from build123d import *

# Parameters (mm, degrees)
SKETCH1_W           = 47
SKETCH1_H           = 17
BOSS_EXTRUDE1_DEPTH = 23
SKETCH2_W           = 4
SKETCH2_H           = 18
CUT_EXTRUDE1_DEPTH  = 38.016888038
SKETCH3_R           = 2
CUT_EXTRUDE2_DEPTH  = 8


with BuildPart() as part:
    # Sketch1 → Boss-Extrude1 (new body)
    with BuildSketch(Plane(origin=(0, 0, 0), x_dir=(1, 0, 0), z_dir=(0, 1, 0))):
        Rectangle(SKETCH1_W, SKETCH1_H)
    extrude(amount=BOSS_EXTRUDE1_DEPTH)

    # Sketch2 → Cut-Extrude1 (cut, through all)
    with BuildSketch(Plane.XY.offset(8.5)):
        with Locations((-20.70480001, 14)):
            Rectangle(SKETCH2_W, SKETCH2_H)
        with Locations((-15.55480001, 14)):
            Rectangle(SKETCH2_W, SKETCH2_H)
        with Locations((-10.40480001, 14)):
            Rectangle(SKETCH2_W, SKETCH2_H)
        with Locations((-5.25480001, 14)):
            Rectangle(SKETCH2_W, SKETCH2_H)
        with Locations((-0.10480001, 14)):
            Rectangle(SKETCH2_W, SKETCH2_H)
        with Locations((5.04519999, 14)):
            Rectangle(SKETCH2_W, SKETCH2_H)
        with Locations((10.19519999, 14)):
            Rectangle(SKETCH2_W, SKETCH2_H)
        with Locations((15.34519999, 14)):
            Rectangle(SKETCH2_W, SKETCH2_H)
        with Locations((20.49519999, 14)):
            Rectangle(SKETCH2_W, SKETCH2_H)
    extrude(amount=-CUT_EXTRUDE1_DEPTH, mode=Mode.SUBTRACT)

    # Sketch3 → Cut-Extrude2 (cut)
    with BuildSketch(Plane.XZ):
        with Locations(Location((-20.600691388, 0, 0), (0, 0, 270))):
            Circle(SKETCH3_R)
        with Locations(Location((20.600691388, 0, 0), (0, 0, 341.307868808))):
            Circle(SKETCH3_R)
    extrude(amount=-CUT_EXTRUDE2_DEPTH, mode=Mode.SUBTRACT)


solid = part.part
Can you work these out from the model? Positions are in its coordinate system, mm. A direction names the side the tool comes from. Coordinates: 2 decimals unless noted, no trailing zeros. Loops run counter-clockwise (first coordinate to the right, second up) from the corner with the lowest first, then second, coordinate; pieces in that order, holes last. Notation, with made-up numbers: (-23, -23.75) - (23, -23.75) arc R31 cw to (23, 11.25) - close; hole circle Ø5 at (-2, 18.5). An arc over 180 degrees is marked (long way). Put each result on its own line as item: value. Start each with the question number.
Item 1: Suppose I cut it at D-D (y = 2.75). Please give me the cut outline in (x, z).
Item 2: If I drill on line 1 along X through (y, z) = (2.75, 0); line 2 along Y through (x, z) = (0, -5.5), over which ranges is the centre line in solid material (lowest first)?
Item 3: For pin 1 (1 mm diameter, centred on x = 0, y = 18.5, fed in from -Z); pin 2 (1.2 mm diameter, centred on x = 4.5, z = -1.5, fed in from +Y), each with a flat end and sliding along its axis, tell me the tip position at first contact or that it passes through.
Item 4: Which directions (+Z, -Z, +X, -X, +Y, -Y) give clear straight access to the entire face, cutting with the end or side of a thin tool? Please do faces 4 (the face through (10, 5, 0)), 5 (the face through (23, 23, 0)).
Item 5: Suppose I cut it at A-A (y = 18.5). State how many separate pieces and enclosed holes the cut face has, and give its area (3 significant figures).
Item 6: If we mould it in two halves opening along X, with no side actions, what happens to faces 1 (the face through (-23.5, 11, 0)), 2 (the face through (0, 4, -8.5)), 3 (the face through (-7.255, 14, 0))? For each: +X half, -X half, draft (parallel to the pull), parting line (faces both ways), or undercut.
Item 7: Suppose I cut it at B-B (x = 9). Please give me the cut outline in (y, z).
Here are the results:
1. outline: (-23.5, -8.5) - (23.5, -8.5) - (23.5, 8.5) - (-23.5, 8.5) - close; hole circle Ø4 at (-20.6, 0); hole circle Ø4 at (20.6, 0)
2. line 1: -23.5 to -22.6, -18.6 to 18.6, 22.6 to 23.5
2. line 2: 0 to 5
3. pin 1: through
3. pin 2: y = 5
4. face 4: +Z, -Z, +Y
4. face 5: +Z, -Z, +X, -X, +Y
5. separate pieces: 10
5. enclosed holes: 0
5. area: 187 mm²
6. face 1: -X half
6. face 2: draft
6. face 3: undercut
7. outline: (0, -8.5) - (5, -8.5) - (5, 8.5) - (0, 8.5) - close
